Autodesk Inventor part; units mm, degrees
ref_plane "YZ Plane" through (0, 0, 0) normal (1, 0, 0) x (0, 1, 0)
ref_plane "XZ Plane" through (0, 0, 0) normal (0, 1, 0) x (-1, 0, 0)
ref_plane "XY Plane" through (0, 0, 0) normal (0, 0, 1) x (1, 0, 0)
sketch "Sketch1" plane through (0, 0, 0) normal (0, 0, 1) x (1, 0, 0)
  point P0 (0, 0)
sketch "Sketch2" plane through (0, 0, 0) normal (0, 1, 0) x (-1, 0, 0)
  line L0 (0, 0) -> (-330, 0)
  line L1 (-330, 0) -> (-330, 80)
  line L2 (-330, 80) -> (0, 80)
  line L3 (0, 80) -> (0, 0)
  dimension "d0" = 330
  dimension "d1" = 80
extrude "Extrusion1" add sketch "Sketch2" along normal blind 2
sketch "Sketch3" plane through (0, 2, 0) normal (0, 1, 0) x (1, 0, 0)
  line L0 (0, 0) -> (0, -80)
  line L1 (330, -80) -> (330, 0)
  line L2 (0, -39) -> (0, -41)
  line L3 (330, -39) -> (330, -41)
  line L4 (165, -39) -> (65, -39)
  line L5 (65, -39) -> (65, -41)
  line L6 (65, -41) -> (265, -41)
  line L7 (265, -41) -> (265, -39)
  line L8 (165, -39) -> (265, -39)
  dimension "d5" = 165
  dimension "d6" = 100
  dimension "d7" = 2
  dimension "d8" = 200
extrude "Extrusion2" add sketch "Sketch3" along normal blind 20
sketch "Sketch4" plane through (65, 2, 41) normal (0, 0, 1) x (1, 0, 0)
  circle A0 centre (100, 10) radius 7.5
  circle A1 centre (12.5, 10) radius 7.5
  circle A2 centre (187.5, 10) radius 7.5
  point P0 (-65, -2)
  dimension "d11" = 15
  dimension "d12" = 15
  dimension "d13" = 15
extrude "Extrusion3" cut sketch "Sketch4" against normal through all
sketch "Sketch5" plane through (0, 0, 0) normal (0, -1, 0) x (1, 0, 0)
  line L0 (0, 80) -> (330, 80)
  line L1 (10, 0) -> (12, 0)
  line L2 (12, 0) -> (12, 80)
  line L3 (12, 80) -> (10, 80)
  line L4 (10, 80) -> (10, 0)
  line L5 (330, 0) -> (0, 0)
  line L6 (320, 0) -> (318, 0)
  line L7 (318, 0) -> (318, 80)
  line L8 (318, 80) -> (320, 80)
  line L9 (320, 80) -> (320, 0)
  dimension "d16" = 2
  dimension "d17" = 2
extrude "Extrusion4" add sketch "Sketch5" along normal blind 30 contours L0 L2 L1 L4 | L0 L9 L5 L7
sketch "Sketch6" plane through (10, 0, 0) normal (-1, 0, 0) x (0, 0, 1)
  circle A0 centre (70, -15) radius 7.5
  point P0 (0, 0)
  dimension "d23" = 15
extrude "Extrusion5" add sketch "Sketch6" against normal blind 310
sketch "Sketch7" plane through (10, 0, 0) normal (-1, 0, 0) x (0, 0, 1)
  circle A0 centre (10, -15) radius 7.5
  point P0 (0, 0)
  dimension "d26" = 15
extrude "Extrusion6" cut sketch "Sketch7" against normal through all
properties part number "Claw_Platform_2"
Read the model definition and answer for the solid it produces. Units are mm, in the model's axes. A direction names the side the tool comes from. Coordinates: 2 decimals unless noted, no trailing zeros. Loops run counter-clockwise (first coordinate to the right, second up) from the corner with the lowest first, then second, coordinate; pieces in that order, holes last.
(1) The part is cut by section A-A (x = 165). Determine the outline of the cut face in (y, z), and give its area (3 significant figures).
Solution:
outline: circle Ø15 at (-15, 70); (0, 0) - (2, 0) - (2, 39) - (4.5, 39) - (4.5, 41) - (2, 41) - (2, 80) - (0, 80) - close; (19.5, 39) - (22, 39) - (22, 41) - (19.5, 41) - close
area: 347 mm2
(2) The part is cut by section D-D (x = 293). Determine the outline of the cut face in (y, z), and give its area (3 significant figures).
Solution:
outline: circle Ø15 at (-15, 70); (0, 0) - (2, 0) - (2, 80) - (0, 80) - close
area: 337 mm2
(3) A tool of negligible diameter and unlimited length cuts with its end or side. For faces 4 (the face through (320, -15, 41)), 5 (the face through (167, 0, 41)), 6 (the face through (164, 21, 41)), 7 (the face through (162.858, -14.67, 62.507)), 8 (the face through (166, 21, 39)), from which of +Z, -Z, +X, -X, +Y, -Y can it reach the whole face along a straight path? Write none if from no direction.
Solution:
face 4: +Z, -Z, +X, -Y
face 5: +Z, -Z
face 6: +Z, +X, -X, +Y
face 7: none
face 8: -Z, +X, -X, +Y
(4) The part is cut by section B-B (y = -15). Determine the outline of the cut face in (x, z), and give its area (3 significant figures).
Solution:
outline: (10, 0) - (12, 0) - (12, 2.5) - (10, 2.5) - close; (10, 17.5) - (12, 17.5) - (12, 62.5) - (318, 62.5) - (318, 17.5) - (320, 17.5) - (320, 80) - (318, 80) - (318, 77.5) - (12, 77.5) - (12, 80) - (10, 80) - close; (318, 0) - (320, 0) - (320, 2.5) - (318, 2.5) - close
area: 4,850 mm2
(5) The part is cut by section C-C (z = 10). Determine the outline of the cut face in (x, y), and give its area (3 significant figures).
Solution:
outline: (0, 0) - (10, 0) - (10, -7.5) - (12, -7.5) - (12, 0) - (318, 0) - (318, -7.5) - (320, -7.5) - (320, 0) - (330, 0) - (330, 2) - (0, 2) - close; (10, -30) - (12, -30) - (12, -22.5) - (10, -22.5) - close; (318, -30) - (320, -30) - (320, -22.5) - (318, -22.5) - close
area: 720 mm2
(6) Consider line 1 along Y through (x, z) = (252, 40); line 2 along Y through (x, z) = (319, 10); line 3 along X through (y, z) = (-21, 19). Determine where each line is inside the solid, lowest interval first.
Solution:
line 1: y = 0 to 4.52, 19.48 to 22
line 2: y = -30 to -22.5, -7.5 to 2
line 3: x = 10 to 12, 318 to 320
(7) The mould has two halves that part along Z. Classify faces 1 (the face through (164, 1, 0)), 2 (the face through (10.986, -14.67, 2.507)), 3 (the face through (10, -15, 39)): released by +Z, released by -Z, zero draft, split by the parting line, or undercut.
Solution:
face 1: released by -Z
face 2: undercut
face 3: zero draft
(8) Flat-ended cylindrical pins translate along their axes: pin 1 Ø24 at (y, z) = (-15, 10) entering from +X; pin 2 Ø3 at (x, z) = (171, 27.5) entering from +Y; pin 3 Ø12 at (y, z) = (12.5, 67.5) entering from +X; pin 4 Ø15 at (y, z) = (-18, 42) entering from -X. Find the tip coordinate at first contact, or state that the pin passes through.
Solution:
pin 1: stops at x = 320
pin 2: stops at y = 2
pin 3: passes through
pin 4: stops at x = 10
